Autodesk Inventor part; units mm, degrees
ref_plane "YZ Plane" through (0, 0, 0) normal (1, 0, 0) x (0, 1, 0)
ref_plane "XZ Plane" through (0, 0, 0) normal (0, 1, 0) x (-1, 0, 0)
ref_plane "XY Plane" through (0, 0, 0) normal (0, 0, 1) x (1, 0, 0)
sketch "スケッチ1" plane through (0, 0, 0) normal (1, 0, 0) x (0, 1, 0)
  line L0 (0, 0) -> (15, 0)
  line L1 (7.5, 0) -> (7.5, 100)
  arc A0 (6.5, 100) -> (0, 0) centre (699.9841, 4.7123) ccw
  arc A1 (15, 0) -> (8.5, 100) centre (-684.9841, 4.7123) ccw
  line L2 (6.5, 100) -> (8.5, 100)
  dimension "d0" = 15
  dimension "d1" = 100
  dimension "d3" = 700
  dimension "d4" = 700
extrude "押し出し1" add sketch "スケッチ1" against normal blind 2
chamfer "面取り1" distance 2 angle 45 1 edges at (0, 13.5418, 50.1165)
sketch "スケッチ2" plane through (0, 0, 0) normal (1, 0, 0) x (0, 0, -1)
  circle A0 centre (-5, 7.5) radius 1.7
  point P0 (0, 0)
  dimension "d10" = 3.4
extrude "押し出し2" cut sketch "スケッチ2" against normal blind 2
properties part number "scissor" material "ステンレス鋼"
For this review, take the finished solid that the model builds, in its own axes (mm). Give positions to 0.01 mm unless a question says otherwise; leave off trailing zeros. Write each loop counter-clockwise with the first axis right and the second up, starting at its lowest first coordinate (ties: lowest second). Pieces come first, ordered by that corner, then holes. Notation, with made-up numbers: M 12.25,-8.5 L 60.25,-8.5 A14 ccw 60.25,12.5 Z; hole C 51,-23.75 d5. An arc over 180 degrees is marked long. Answer as a JSON object with one key per item and string values. Group by question number.
Item 1: Consider section B-B on y = 3.5. Write out the cut boundary in (x, z).
Item 2: For probe 1 along Y at (x, z) = (-1.4, 5); probe 2 along Y at (x, z) = (-0.6, 5); probe 3 along X at (y, z) = (14, 33.5), list the stretches that pass through material, from the lowest coordinate up. Write a range as [from, to].
Item 3: Draft analysis for pull direction Y (two halves, no side actions). For faces 1 (the conical face through (-0.79, 12.28, 50.87)), 2 (the cylindrical face through (-1, 6, 4.2)), 3 (the flat face through (-2, 7, 40)), 4 (the cylindrical face through (-0.986, 1.504, 50.817)), state which applies: +Y half, -Y half, draft (parallel to the pull), parting line (faces both ways), or undercut.
Item 4: Consider section A-A on x = -0.4. Write out the cut boundary in (y, z).
Check result:
{
 "1": {"outline": "M -2,0 L 0,0 L 0,74.78 L -2,74.78 Z"},
 "2": {"probe 1": "y = [-0.02, 5.8], [9.2, 14.42]", "probe 2": "y = [-0.02, 5.8], [9.2, 13.62]", "probe 3": "x = [-2, -1.58]"},
 "3": {"face 1": "+Y half", "face 2": "undercut", "face 3": "draft", "face 4": "-Y half"},
 "4": {"outline": "M 0,0 L 13.4,0 A698.4 ccw 6.89,100 L 6.5,100 A700 ccw Z; hole C 7.5,5 d3.4"}
}
